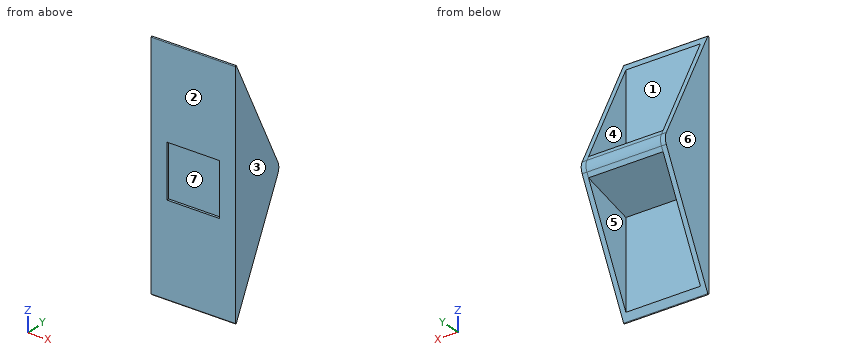
```python
from build123d import *

# Parameters (mm, degrees)
BOSS_EXTRUDE5_DEPTH = 35
SHELL8_T            = -2
BOSS_EXTRUDE6_DEPTH = 31
BOSS_EXTRUDE7_DEPTH = 31
FILLET1_R           = 5
FILLET2_R           = 0.3
FILLET3_R           = 0.3
SKETCH3_W           = 11
SKETCH3_H           = 22
CUT_EXTRUDE2_DEPTH  = 1


with BuildPart() as part:
    # Sketch2 → Boss-Extrude5 (new body)
    with BuildSketch(Plane(origin=(0, 0, 0), x_dir=(0, 0, -1), z_dir=(1, 0, 0))):
        Polygon((0, 0), (50, 0), (0, 25), align=None)
    boss_extrude5 = extrude(amount=BOSS_EXTRUDE5_DEPTH)

    # Mirror1: Boss-Extrude5 across Front Plane
    add(boss_extrude5.mirror(Plane.XY))

    # Shell8
    shell8_openings = [part.faces().sort_by_distance(p)[0] for p in [
        (17.5, 12.5, 25),
        (17.5, 12.5, -25),
    ]]
    offset(amount=SHELL8_T, openings=shell8_openings, kind=Kind.INTERSECTION)

    # 3DSketch9 → Boss-Extrude6 (add)
    with BuildSketch(Plane(origin=(33, 25, 0), x_dir=(0, -0.9850310317593959, -0.1723771054143217), z_dir=(-1, 0, 0))):
        Polygon((0, 0), (2.676141178, -3.617771192), (23.349518196, 0), (21.961909265, 7.929346849), (1.288532246, 4.311575657), align=None)
    extrude(amount=BOSS_EXTRUDE6_DEPTH)

    # 3DSketch10 → Boss-Extrude7 (add)
    with BuildSketch(Plane(origin=(33, 2, -4.024922359), x_dir=(0, 0.9336773848792517, 0.3581152621224651), z_dir=(1, 0, 0))):
        Polygon((0, 0), (-2.139766495, -5.578794866), (19.595590361, -7.515957966), align=None)
        Polygon((2.882772252, 7.515957966), (5.022538747, 13.094752832), (22.478362612, 0), align=None)
    extrude(amount=-BOSS_EXTRUDE7_DEPTH)

    # Fillet1
    fillet1_edges = [part.edges().sort_by_distance(p)[0] for p in [
        (17.5, 25, 0),
    ]]
    fillet(fillet1_edges, radius=FILLET1_R)

    # Fillet2
    fillet2_edges = [part.edges().sort_by_distance(p)[0] for p in [
        (17.5, 0, -50),
    ]]
    fillet(fillet2_edges, radius=FILLET2_R)

    # Fillet3
    fillet3_edges = [part.edges().sort_by_distance(p)[0] for p in [
        (17.5, 0, 50),
    ]]
    fillet(fillet3_edges, radius=FILLET3_R)

    # Sketch3 → Cut-Extrude2 (cut)
    with BuildSketch(Plane.XZ):
        with Locations((12, 0)):
            Rectangle(SKETCH3_W, SKETCH3_H)
        with Locations((23, 0)):
            Rectangle(SKETCH3_W, SKETCH3_H)
    extrude(amount=-CUT_EXTRUDE2_DEPTH, mode=Mode.SUBTRACT)


solid = part.part
```
Could you check a few things on this model? Use its own coordinates, in mm. Face numbers are marked on the shaded views. A direction names the side the tool comes from. Round coordinates to 2 decimals unless told otherwise and drop trailing zeros. Loops run counter-clockwise (first coordinate to the right, second up) from the corner with the lowest first, then second, coordinate; pieces in that order, holes last.
Q1. Please list where these lines run through material, in increasing order: L1, parallel to X at y = 12.5, z = 23; L2, parallel to Y at x = 19, z = -38; L3, parallel to Z at x = 20.5, y = 2.75.
Q2. I want a section at B-B (x = 14.5). Write out the boundary of the cut face in (y, z).
Q3. Thinking about a two-plate mould opening in X: for the marked faces 1, 2 and 3, which applies, pulls with the +X half, pulls with the -X half, needs draft (parallel to the pull), parting line crosses it, or undercut?
Q4. I want a section at D-D (z = 0). Write out the boundary of the cut face in (x, y).
Q5. I want a section at A-A (z = -24). Write out the boundary of the cut face in (x, y), and give its area (3 significant figures).
Q6. On a 3-axis mill with a long thin cutter (end or side, diameter ignored), from which of +Z, -Z, +X, -X, +Y, -Y can I reach the whole of each face in a straight line? I mean the marked faces 4, 5, 6 and 7. Say none if no direction works.
Q7. I want a section at C-C (y = 9.75). Write out the boundary of the cut face in (x, z), and give its area (3 significant figures).
Q8. For P1, Ø10, axis at x = 11, y = 20.5, coming from the -Z side; P2, Ø12, axis at x = 12, z = -37.5, coming from the +Y side; P3, Ø6.5, axis at x = 18, z = -2.5, coming from the -Y side, each with a flat end and sliding along its axis, tell me the tip position at first contact or that it passes through.
Answer below:
1. L1: x = 0 to 2, 33 to 35
1. L2: y = 0 to 2
1. L3: z = -9.79 to 9.79
2. outline: (0, -48.73) arc R0.3 ccw to (0.57, -48.86) - (2, -46) - (2, -10) - (22.99, -4.02) - (23.88, -2.24) arc R5 ccw to (23.88, 2.24) - (22.99, 4.02) - (2, 10) - (2, 46) - (0.57, 48.86) arc R0.3 ccw to (0, 48.73) - (0, 11) - (1, 11) - (1, -11) - (0, -11) - close
3. face 1: undercut
3. face 2: needs draft
3. face 3: pulls with the +X half
4. outline: (0, 0) - (6.5, 0) - (6.5, 1) - (28.5, 1) - (28.5, 0) - (35, 0) - (35, 24.41) - (0, 24.41) - close
5. outline: (0, 0) - (35, 0) - (35, 13) - (33, 13) - (33, 2) - (2, 2) - (2, 13) - (0, 13) - close
5. area: 114 mm2
6. face 4: +Z, +Y
6. face 5: -Z, +Y
6. face 6: +Z, -Z, -X, +Y, -Y
6. face 7: -Y
7. outline: (0, -30.5) - (2, -30.5) - (2, -7.79) - (33, -7.79) - (33, -30.5) - (35, -30.5) - (35, 30.5) - (33, 30.5) - (33, 7.79) - (2, 7.79) - (2, 30.5) - (0, 30.5) - close
7. area: 727 mm2
8. P1: stops at z = -6.16
8. P2: stops at y = 2
8. P3: stops at y = 1
